Read the model definition and answer for the solid it produces. Units are mm, in the model's axes. Face numbers are marked on the shaded views. Round coordinates to 2 decimals unless told otherwise and drop trailing zeros. Loops run counter-clockwise (first coordinate to the right, second up) from the corner with the lowest first, then second, coordinate; pieces in that order, holes last. Notation, with made-up numbers: M 74,32 L 104,32 A32 ccw 104,69 Z; hole C 10.25,37.25 d1. An arc over 180 degrees is marked long. Answer as CSV lines item,"result".
```python
from build123d import *

# Parameters (mm, degrees)
F1_DEPTH = 25.4
F3_D     = 20.32
F5_D     = 22.86


with BuildPart() as f1:
    # F0 (on Front) → F1 (new body)
    with BuildSketch(Plane.XZ):
        with BuildLine():
            Line((37.473018, -16.239311), (37.473018, 16.239311))
            ThreePointArc((37.473018, 16.239311), (21.421916, 0), (37.473018, -16.239311))
        make_face()
        with BuildLine():
            ThreePointArc((53.902746, 0), (49.07891, 11.550446), (37.473018, 16.239311))
            Line((37.473018, 16.239311), (37.473018, -16.239311))
            ThreePointArc((37.473018, -16.239311), (49.07891, -11.550446), (53.902746, 0))
        make_face()
        with BuildLine():
            ThreePointArc((-42.453576, 15.307551), (-31.629503, 10.824073), (-27.146025, 0))
            ThreePointArc((-27.146025, 0), (-31.629503, -10.824073), (-42.453576, -15.307551))
            Line((-42.453576, -15.307551), (37.473018, -16.239311))
            ThreePointArc((37.473018, -16.239311), (21.421916, 0), (37.473018, 16.239311))
            Line((37.473018, 16.239311), (-42.453576, 15.307551))
        make_face()
        with BuildLine():
            ThreePointArc((-42.453576, -15.307551), (-31.629503, -10.824073), (-27.146025, 0))
            ThreePointArc((-27.146025, 0), (-31.629503, 10.824073), (-42.453576, 15.307551))
            Line((-42.453576, 15.307551), (-42.810429, -15.303391))
            Line((-42.810429, -15.303391), (-42.453576, -15.307551))
        make_face()
        with BuildLine():
            Line((-42.810429, -15.303391), (-42.453576, 15.307551))
            ThreePointArc((-42.453576, 15.307551), (-57.760087, 0.178439), (-42.810429, -15.303391))
        make_face()
    extrude(amount=F1_DEPTH)

    # F3 (through all)
    with Locations(Plane(origin=(0, 0, 0), x_dir=(1, 0, 0), z_dir=(0, 1, 0))):
        with Locations((-30.845791, 0), (30.270591, 0)):
            Hole(F3_D / 2)

    # F5 (through all)
    with Locations(Plane(origin=(0, 0, 0), x_dir=(-1, 0, 0), z_dir=(0, 1, 0))):
        with Locations((0, 0)):
            Hole(F5_D / 2)


solid = f1.part
```
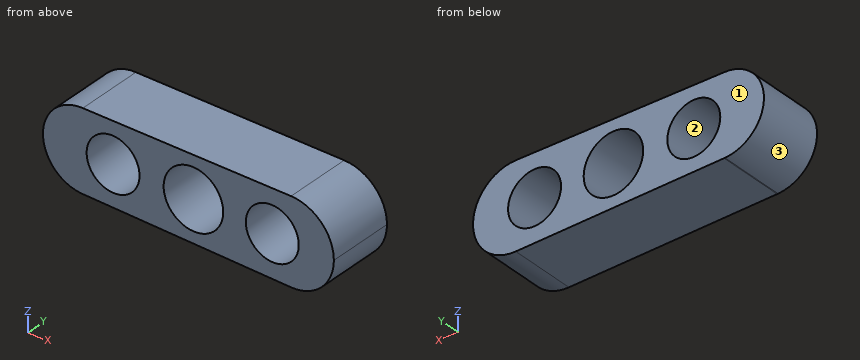
1) Find section D-D, the plane x = 4.5. Give the vertices of the cut face in (y, z).
Evaluation:
outline,"M -25.4,-15.85 L 0,-15.85 L 0,-10.51 L -25.4,-10.51 Z; M -25.4,10.51 L 0,10.51 L 0,15.85 L -25.4,15.85 Z"
2) Find section C-C, the plane z = -1.5. Give the vertices of the cut face in (x, y), then the cut area to 3 significant figures.
Evaluation:
outline,"M -57.69,-25.4 L -40.89,-25.4 L -40.89,0 L -57.69,0 Z; M -20.8,-25.4 L -11.33,-25.4 L -11.33,0 L -20.8,0 Z; M 11.33,-25.4 L 20.22,-25.4 L 20.22,0 L 11.33,0 Z; M 40.32,-25.4 L 53.83,-25.4 L 53.83,0 L 40.32,0 Z"
area,"1,240 mm^2"
3) Each of these flat-tipped pins is pushed along its axis until it touches: P1, Ø1.5, axis at x = -36.5, y = -9, coming from the +Z side; P2, Ø16.5, axis at x = 30.27, z = 0, coming from the -Y side; P3, Ø10, axis at x = 5.5, y = -17, coming from the +Z side; P4, Ø10, axis at y = -17, z = 8, coming from the +X side. Where does it stop, or does it pass through?
Evaluation:
P1,"stops at z = 15.39"
P2,"passes through"
P3,"stops at z = 15.92"
P4,"stops at x = 53.62"
4) Find section B-B, the plane y = -2. Give the vertices of the cut face in (x, z).
Evaluation:
outline,"M -42.81,-15.3 L -42.45,-15.31 L 37.47,-16.24 A16.24 ccw long 37.47,16.24 L -42.45,15.31 A15.31 ccw Z; hole C -30.85,0 d20.32; hole C 0,0 d22.86; hole C 30.27,0 d20.32"
5) Find section A-A, the plane x = -24. Give the vertices of the cut face in (y, z).
Evaluation:
outline,"M -25.4,-15.52 L 0,-15.52 L 0,-7.51 L -25.4,-7.51 Z; M -25.4,7.51 L 0,7.51 L 0,15.52 L -25.4,15.52 Z"
6) Determine the mould class of the marked faces 1, 2 and 3 for opening direction Z: released by +Z, released by -Z, zero draft, split by the parting line, or undercut.
Evaluation:
face 1,"zero draft"
face 2,"undercut"
face 3,"split by the parting line"
7) Straight lines are drawn through the part: line 1 (X direction, y = -4.75, z = 1.5); line 2 (X direction, y = -2, z = 2.5); line 3 (Z direction, x = 0, y = -6). For each, find the intervals that lie inside material, in ascending order.
Evaluation:
line 1,"x = -57.69 to -40.89, -20.8 to -11.33, 11.33 to 20.22, 40.32 to 53.83"
line 2,"x = -57.56 to -40.69, -21 to -11.15, 11.15 to 20.42, 40.12 to 53.71"
line 3,"z = -15.8 to -11.43, 11.43 to 15.8"
